Verification items for this drawing (mm, ordinates from the low corner). Round coordinates to 2 decimals unless told otherwise and drop trailing zeros. Loops run counter-clockwise (first coordinate to the right, second up) from the corner with the lowest first, then second, coordinate; pieces in that order, holes last. Notation, with made-up numbers: (27.5, -27) -> (67.5, -27) arc R28 cw to (67.5, 3) -> close; hole circle Ø8 at (-8.5, 56.25). An arc over 180 degrees is marked (long way). One line per item, written item: value. Start each with the question number.
1. Go/stop test with flat-tipped pins: pin 1 (5 mm diameter, centred on y = 19, z = 23.5, fed in from -X) (1 decimal); pin 2 (1.5 mm diameter, centred on y = 4, z = 38.5, fed in from -X) (1 decimal); pin 3 (3 mm diameter, centred on y = 11, z = 110, fed in from -X). Record where each tip stops, or that it passes through.
2. Cross-section at A-A on x = 184.15. Record the cut outline in (y, z).
3. Material ranges on L1, parallel to Z at x = 31.75, y = 13; L2, parallel to X at y = 19.75, z = 66; L3, parallel to Z at x = 175, y = 11.5, recorded low to high.
4. Cross-section at B-B on z = 63.5. Record the cut outline in (x, y).
5. Cross-section at D-D on y = 17.5. Record the cut outline in (x, z), then the cut area to 3 significant figures.
6. Release check for a two-part mould opening along X. For the marked faces 1, 2 and 3 record: +X half, -X half, draft (parallel to the pull), parting line (faces both ways), or undercut.
7. Cross-section at C-C on z = 81.5. Record the cut outline in (x, y) (1 decimal), then the cut area to 4 significant figures.
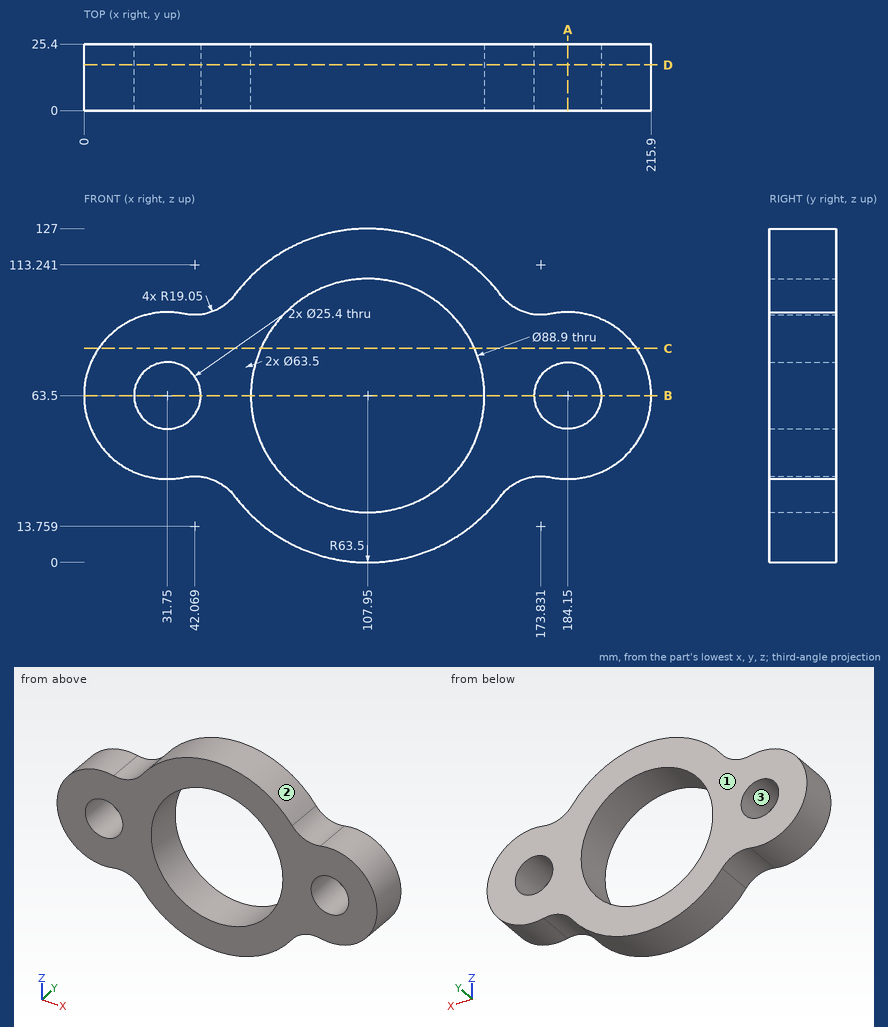
Taken from the geometry:
1. pin 1: stops at x = 56.7
1. pin 2: stops at x = 11.3
1. pin 3: stops at x = 63.15
2. outline: (0, 31.75) -> (25.4, 31.75) -> (25.4, 50.8) -> (0, 50.8) -> close; (0, 76.2) -> (25.4, 76.2) -> (25.4, 95.25) -> (0, 95.25) -> close
3. L1: z = 31.75 to 50.8, 76.2 to 95.25
3. L2: x = 0.1 to 19.3, 44.2 to 63.57, 152.33 to 171.7, 196.6 to 215.8
3. L3: z = 32.77 to 54.69, 72.31 to 94.23
4. outline: (0, 0) -> (19.05, 0) -> (19.05, 25.4) -> (0, 25.4) -> close; (44.45, 0) -> (63.5, 0) -> (63.5, 25.4) -> (44.45, 25.4) -> close; (152.4, 0) -> (171.45, 0) -> (171.45, 25.4) -> (152.4, 25.4) -> close; (196.85, 0) -> (215.9, 0) -> (215.9, 25.4) -> (196.85, 25.4) -> close
5. outline: (38.2, 32.41) arc R19.05 cw to (57.27, 25.24) arc R63.5 ccw to (158.63, 25.24) arc R19.05 cw to (177.7, 32.41) arc R31.75 ccw (long way) to (177.7, 94.59) arc R19.05 cw to (158.63, 101.76) arc R63.5 ccw to (57.27, 101.76) arc R19.05 cw to (38.2, 94.59) arc R31.75 ccw (long way) to start; hole circle Ø25.4 at (31.75, 63.5); hole circle Ø88.9 at (107.95, 63.5); hole circle Ø25.4 at (184.15, 63.5)
5. area: 10,600 mm2
6. face 1: draft
6. face 2: parting line
6. face 3: undercut
7. outline: (5.6, 0) -> (67.3, 0) -> (67.3, 25.4) -> (5.6, 25.4) -> close; (148.6, 0) -> (210.3, 0) -> (210.3, 25.4) -> (148.6, 25.4) -> close
7. area: 3,135 mm2
